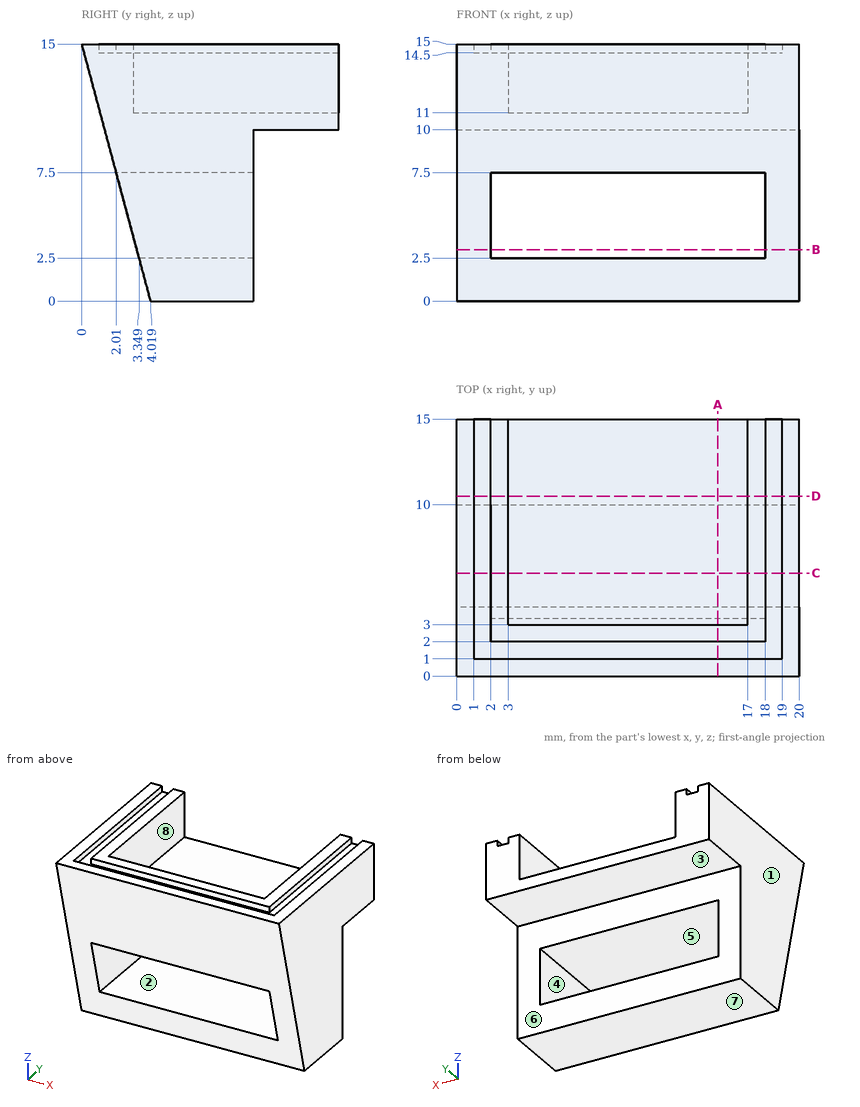
Answer from the drawing. Dimensions are ordinates in mm from the lowest x, y and z of the part. A direction names the side the tool comes from. Round coordinates to 2 decimals unless told otherwise and drop trailing zeros. Loops run counter-clockwise (first coordinate to the right, second up) from the corner with the lowest first, then second, coordinate; pieces in that order, holes last.
Q1. Each of these flat-tipped pins is pushed along its axis until it touches: pin 1 (7.5 mm diameter, centred on x = 7, y = 7, fed in from +Z); pin 2 (8 mm diameter, centred on x = 14, z = 3, fed in from +Y); pin 3 (4 mm diameter, centred on x = 11, y = 12.5, fed in from -Z). Where does it stop, or does it pass through?
Q2. Consider probe 1 along X at (y, z) = (5, 2.75); probe 2 along Z at (x, y) = (12.75, 7.5); probe 3 along Z at (x, y) = (2.75, 7.25). Determine where each line is inside the solid, lowest interval first.
Q3. Section B-B on z = 3 is taken. Write down the section's boundary in (x, y) (1 decimal).
Q4. Section D-D on y = 10.5 is taken. Write down the section's boundary in (x, z), and give its area (3 significant figures).
Q5. Section A-A on x = 15.25 is taken. Write down the section's boundary in (y, z).
Q6. Which of the six approach directions +Z, -Z, +X, -X, +Y, -Y give full straight-line access (tool end or side, diameter ignored) to the marked faces 5, 6, 7 and 8?
Q7. Determine the mould class of the marked faces 1, 2, 3 and 4 for opening direction Z: released by +Z, released by -Z, zero draft, split by the parting line, or undercut.
Q8. Section C-C on y = 6 is taken. Write down the section's boundary in (x, z).
Output:
1. pin 1: stops at z = 11
1. pin 2: stops at y = 10
1. pin 3: stops at z = 10
2. probe 1: x = 0 to 2, 18 to 20
2. probe 2: z = 0 to 2.5, 7.5 to 11
2. probe 3: z = 0 to 2.5, 7.5 to 15
3. outline: (0, 3.2) - (2, 3.2) - (2, 10) - (0, 10) - close; (18, 3.2) - (20, 3.2) - (20, 10) - (18, 10) - close
4. outline: (0, 10) - (20, 10) - (20, 15) - (19, 15) - (19, 14.5) - (18, 14.5) - (18, 15) - (17, 15) - (17, 11) - (3, 11) - (3, 15) - (2, 15) - (2, 14.5) - (1, 14.5) - (1, 15) - (0, 15) - close
4. area: 43.0 mm2
5. outline: (0, 15) - (2.01, 7.5) - (10, 7.5) - (10, 10) - (15, 10) - (15, 11) - (3, 11) - (3, 15) - (2, 15) - (2, 14.5) - (1, 14.5) - (1, 15) - close; (3.35, 2.5) - (4.02, 0) - (10, 0) - (10, 2.5) - close
6. face 5: +Y, -Y
6. face 6: -Z, +X, -X, +Y
6. face 7: -Z, +X, -X, +Y, -Y
6. face 8: +Z, +Y
7. face 1: zero draft
7. face 2: undercut
7. face 3: released by -Z
7. face 4: undercut
8. outline: (0, 0) - (20, 0) - (20, 15) - (19, 15) - (19, 14.5) - (18, 14.5) - (18, 15) - (17, 15) - (17, 11) - (3, 11) - (3, 15) - (2, 15) - (2, 14.5) - (1, 14.5) - (1, 15) - (0, 15) - close; hole (2, 2.5) - (18, 2.5) - (18, 7.5) - (2, 7.5) - close
